The model under review builds one solid part; all positions refer to its coordinate system, in mm. A direction names the side the tool comes from. Give positions to 0.01 mm unless a question says otherwise; leave off trailing zeros. Write item = value, one per line.
```python
from build123d import *

# Parameters (mm, degrees)
SKETCH_1_R          = 1.6
SKETCH_1_R_2        = 2.1
SKETCH_1_R_3        = 2
EXTRUDE_1_DEPTH     = 5
SKETCH_2_R          = 2.25
CUT_EXTRUDE_2_DEPTH = 10
SKETCH_3_R          = 2.1
CUT_EXTRUDE_3_DEPTH = 27
CUT_EXTRUDE_4_DEPTH = 20
SKETCH_5_R          = 2.1
CUT_EXTRUDE_5_DEPTH = 20


with BuildPart() as part:
    # 草图1 → 凸台-拉伸1 (new body)
    with BuildSketch(Plane(origin=(0, 0, 0), x_dir=(1, 0, 0), z_dir=(0, 1, 0))):
        with BuildLine():
            Line((-43, -137), (43, -137))
            ThreePointArc((43, -137), (50.071067812, -134.071067812), (53, -127))
            Line((53, -127), (53, 132))
            ThreePointArc((53, 132), (50.071067812, 139.071067812), (43, 142))
            Line((43, 142), (-43, 142))
            ThreePointArc((-43, 142), (-50.071067812, 139.071067812), (-53, 132))
            Line((-53, 132), (-53, -127))
            ThreePointArc((-53, -127), (-50.071067812, -134.071067812), (-43, -137))
        make_face()
        with Locations((-40, 132)):
            Circle(SKETCH_1_R, mode=Mode.SUBTRACT)
        with Locations((-9, 132)):
            Circle(SKETCH_1_R, mode=Mode.SUBTRACT)
        with Locations((-9, 101)):
            Circle(SKETCH_1_R, mode=Mode.SUBTRACT)
        with Locations((-40, 101)):
            Circle(SKETCH_1_R, mode=Mode.SUBTRACT)
        with Locations((9, 101)):
            Circle(SKETCH_1_R, mode=Mode.SUBTRACT)
        with Locations((40, 101)):
            Circle(SKETCH_1_R, mode=Mode.SUBTRACT)
        with Locations((9, 132)):
            Circle(SKETCH_1_R, mode=Mode.SUBTRACT)
        with Locations((40, 132)):
            Circle(SKETCH_1_R, mode=Mode.SUBTRACT)
        with Locations((-37, -112)):
            Circle(SKETCH_1_R_2, mode=Mode.SUBTRACT)
        with Locations((-37, -32)):
            Circle(SKETCH_1_R_2, mode=Mode.SUBTRACT)
        with Locations((-37, 48)):
            Circle(SKETCH_1_R_2, mode=Mode.SUBTRACT)
        with Locations((37, -112)):
            Circle(SKETCH_1_R_2, mode=Mode.SUBTRACT)
        with Locations((37, -32)):
            Circle(SKETCH_1_R_2, mode=Mode.SUBTRACT)
        with Locations((37, 48)):
            Circle(SKETCH_1_R_2, mode=Mode.SUBTRACT)
        with Locations((-40, 91)):
            Circle(SKETCH_1_R_2, mode=Mode.SUBTRACT)
        with Locations((-40, 81)):
            Circle(SKETCH_1_R_2, mode=Mode.SUBTRACT)
        with Locations((-40, 71)):
            Circle(SKETCH_1_R_2, mode=Mode.SUBTRACT)
        with Locations((-40, 61)):
            Circle(SKETCH_1_R_2, mode=Mode.SUBTRACT)
        with Locations((40, 61)):
            Circle(SKETCH_1_R_2, mode=Mode.SUBTRACT)
        with Locations((40, 71)):
            Circle(SKETCH_1_R_2, mode=Mode.SUBTRACT)
        with Locations((40, 81)):
            Circle(SKETCH_1_R_2, mode=Mode.SUBTRACT)
        with Locations((40, 91)):
            Circle(SKETCH_1_R_2, mode=Mode.SUBTRACT)
        with Locations((-42.25, -5.7)):
            Circle(SKETCH_1_R_2, mode=Mode.SUBTRACT)
        with Locations((-23.75, -5.7)):
            Circle(SKETCH_1_R_2, mode=Mode.SUBTRACT)
        with Locations((23.75, -5.7)):
            Circle(SKETCH_1_R_2, mode=Mode.SUBTRACT)
        with Locations((42.25, -5.7)):
            Circle(SKETCH_1_R_2, mode=Mode.SUBTRACT)
        with Locations((-28, 32.95)):
            Circle(SKETCH_1_R_3, mode=Mode.SUBTRACT)
        with Locations((28, 32.95)):
            Circle(SKETCH_1_R_3, mode=Mode.SUBTRACT)
        with BuildLine():
            Line((21, 91.5), (-21, 91.5))
            ThreePointArc((-21, 91.5), (-23.121320344, 90.621320344), (-24, 88.5))
            Line((-24, 88.5), (-24, 54.5))
            ThreePointArc((-24, 54.5), (-23.121320344, 52.378679656), (-21, 51.5))
            Line((-21, 51.5), (21, 51.5))
            ThreePointArc((21, 51.5), (23.121320344, 52.378679656), (24, 54.5))
            Line((24, 54.5), (24, 88.5))
            ThreePointArc((24, 88.5), (23.121320344, 90.621320344), (21, 91.5))
        make_face(mode=Mode.SUBTRACT)
        with BuildLine():
            Line((-36, 37.5), (-32, 37.5))
            ThreePointArc((-32, 37.5), (-31.292893219, 37.207106781), (-31, 36.5))
            Line((-31, 36.5), (-31, 29.5))
            ThreePointArc((-31, 29.5), (-31.292893219, 28.792893219), (-32, 28.5))
            Line((-32, 28.5), (-36, 28.5))
            ThreePointArc((-36, 28.5), (-36.707106781, 28.792893219), (-37, 29.5))
            Line((-37, 29.5), (-37, 36.5))
            ThreePointArc((-37, 36.5), (-36.707106781, 37.207106781), (-36, 37.5))
        make_face(mode=Mode.SUBTRACT)
        with BuildLine():
            Line((-16, 37.5), (-12, 37.5))
            ThreePointArc((-12, 37.5), (-11.292893219, 37.207106781), (-11, 36.5))
            Line((-11, 36.5), (-11, 29.5))
            ThreePointArc((-11, 29.5), (-11.292893219, 28.792893219), (-12, 28.5))
            Line((-12, 28.5), (-16, 28.5))
            ThreePointArc((-16, 28.5), (-16.707106781, 28.792893219), (-17, 29.5))
            Line((-17, 29.5), (-17, 36.5))
            ThreePointArc((-17, 36.5), (-16.707106781, 37.207106781), (-16, 37.5))
        make_face(mode=Mode.SUBTRACT)
        with BuildLine():
            Line((37, 36.5), (37, 29.5))
            ThreePointArc((37, 29.5), (36.707106781, 28.792893219), (36, 28.5))
            Line((36, 28.5), (32, 28.5))
            ThreePointArc((32, 28.5), (31.292893219, 28.792893219), (31, 29.5))
            Line((31, 29.5), (31, 36.5))
            ThreePointArc((31, 36.5), (31.292893219, 37.207106781), (32, 37.5))
            Line((32, 37.5), (36, 37.5))
            ThreePointArc((36, 37.5), (36.707106781, 37.207106781), (37, 36.5))
        make_face(mode=Mode.SUBTRACT)
        with BuildLine():
            Line((17, 36.5), (17, 29.5))
            ThreePointArc((17, 29.5), (16.707106781, 28.792893219), (16, 28.5))
            Line((16, 28.5), (12, 28.5))
            ThreePointArc((12, 28.5), (11.292893219, 28.792893219), (11, 29.5))
            Line((11, 29.5), (11, 36.5))
            ThreePointArc((11, 36.5), (11.292893219, 37.207106781), (12, 37.5))
            Line((12, 37.5), (16, 37.5))
            ThreePointArc((16, 37.5), (16.707106781, 37.207106781), (17, 36.5))
        make_face(mode=Mode.SUBTRACT)
    extrude(amount=EXTRUDE_1_DEPTH)

    # 草图2 → 切除-拉伸2 (cut)
    with BuildSketch(Plane(origin=(0, 0, 0), x_dir=(1, 0, 0), z_dir=(0, 1, 0))):
        with Locations((-43.25, -80.8)):
            Circle(SKETCH_2_R)
        with Locations((43.25, -80.8)):
            Circle(SKETCH_2_R)
        with Locations((-43.25, -18.8)):
            Circle(SKETCH_2_R)
        with Locations((43.25, -18.8)):
            Circle(SKETCH_2_R)
    extrude(amount=CUT_EXTRUDE_2_DEPTH, mode=Mode.SUBTRACT)

    # 草图3 → 切除-拉伸3 (cut)
    with BuildSketch(Plane(origin=(0, 0, 0), x_dir=(1, 0, 0), z_dir=(0, 1, 0))):
        with Locations((2.28, -125.5)):
            Circle(SKETCH_3_R)
        with Locations((48.28, -125.5)):
            Circle(SKETCH_3_R)
        with Locations((24.28, -99.327742623)):
            Circle(SKETCH_3_R)
        with BuildLine():
            Line((37.78, -120.8), (41.78, -120.8))
            ThreePointArc((41.78, -120.8), (42.487106781, -121.092893219), (42.78, -121.8))
            Line((42.78, -121.8), (42.78, -128.8))
            ThreePointArc((42.78, -128.8), (42.487106781, -129.507106781), (41.78, -129.8))
            Line((41.78, -129.8), (37.78, -129.8))
            ThreePointArc((37.78, -129.8), (37.072893219, -129.507106781), (36.78, -128.8))
            Line((36.78, -128.8), (36.78, -121.8))
            ThreePointArc((36.78, -121.8), (37.072893219, -121.092893219), (37.78, -120.8))
        make_face()
        with BuildLine():
            Line((7.78, -120.8), (11.78, -120.8))
            ThreePointArc((11.78, -120.8), (12.487106781, -121.092893219), (12.78, -121.8))
            Line((12.78, -121.8), (12.78, -128.8))
            ThreePointArc((12.78, -128.8), (12.487106781, -129.507106781), (11.78, -129.8))
            Line((11.78, -129.8), (7.78, -129.8))
            ThreePointArc((7.78, -129.8), (7.072893219, -129.507106781), (6.78, -128.8))
            Line((6.78, -128.8), (6.78, -121.8))
            ThreePointArc((6.78, -121.8), (7.072893219, -121.092893219), (7.78, -120.8))
        make_face()
        with BuildLine():
            Line((21.28, -106.8), (27.28, -106.8))
            ThreePointArc((27.28, -106.8), (27.987106781, -107.092893219), (28.28, -107.8))
            Line((28.28, -107.8), (28.28, -111.8))
            ThreePointArc((28.28, -111.8), (27.987106781, -112.507106781), (27.28, -112.8))
            Line((27.28, -112.8), (21.28, -112.8))
            ThreePointArc((21.28, -112.8), (20.572893219, -112.507106781), (20.28, -111.8))
            Line((20.28, -111.8), (20.28, -107.8))
            ThreePointArc((20.28, -107.8), (20.572893219, -107.092893219), (21.28, -106.8))
        make_face()
        with BuildLine():
            Line((21.28, -86.8), (27.28, -86.8))
            ThreePointArc((27.28, -86.8), (27.987106781, -87.092893219), (28.28, -87.8))
            Line((28.28, -87.8), (28.28, -91.8))
            ThreePointArc((28.28, -91.8), (27.987106781, -92.507106781), (27.28, -92.8))
            Line((27.28, -92.8), (21.28, -92.8))
            ThreePointArc((21.28, -92.8), (20.572893219, -92.507106781), (20.28, -91.8))
            Line((20.28, -91.8), (20.28, -87.8))
            ThreePointArc((20.28, -87.8), (20.572893219, -87.092893219), (21.28, -86.8))
        make_face()
        with BuildLine():
            Line((-8.22, -121.8), (-8.22, -128.8))
            ThreePointArc((-8.22, -128.8), (-8.512893219, -129.507106781), (-9.22, -129.8))
            Line((-9.22, -129.8), (-13.22, -129.8))
            ThreePointArc((-13.22, -129.8), (-13.927106781, -129.507106781), (-14.22, -128.8))
            Line((-14.22, -128.8), (-14.22, -121.8))
            ThreePointArc((-14.22, -121.8), (-13.927106781, -121.092893219), (-13.22, -120.8))
            Line((-13.22, -120.8), (-9.22, -120.8))
            ThreePointArc((-9.22, -120.8), (-8.512893219, -121.092893219), (-8.22, -121.8))
        make_face()
    extrude(amount=CUT_EXTRUDE_3_DEPTH, mode=Mode.SUBTRACT)

    # 草图4 → 切除-拉伸4 (cut)
    with BuildSketch(Plane(origin=(0, 0, 0), x_dir=(1, 0, 0), z_dir=(0, 1, 0))):
        with BuildLine():
            Line((36, -95), (42, -95))
            ThreePointArc((42, -95), (44.121320344, -95.878679656), (45, -98))
            Line((45, -98), (45, -104))
            ThreePointArc((45, -104), (44.121320344, -106.121320344), (42, -107))
            Line((42, -107), (36, -107))
            ThreePointArc((36, -107), (33.878679656, -106.121320344), (33, -104))
            Line((33, -104), (33, -98))
            ThreePointArc((33, -98), (33.878679656, -95.878679656), (36, -95))
        make_face()
    extrude(amount=CUT_EXTRUDE_4_DEPTH, mode=Mode.SUBTRACT)

    # 草图5 → 切除-拉伸5 (cut)
    with BuildSketch(Plane(origin=(0, 0, 0), x_dir=(1, 0, 0), z_dir=(0, 1, 0))):
        with Locations((0, -2)):
            Circle(SKETCH_5_R)
        with Locations((-8, -102)):
            Circle(SKETCH_5_R)
        with Locations((8, -102)):
            Circle(SKETCH_5_R)
    extrude(amount=CUT_EXTRUDE_5_DEPTH, mode=Mode.SUBTRACT)


solid = part.part
```
1. Draft analysis for pull direction Z (two halves, no side actions). For faces 3 (the flat face through (24, 2, 106.8)), 4 (the flat face through (-53, 2, -4)), state which applies: +Z half, -Z half, draft (parallel to the pull), parting line (faces both ways), or undercut.
Findings below:
face_3 = undercut
face_4 = draft
2. Machinability: for faces 1 (the flat face through (24, 2, -71)), 2 (the flat face through (53, 2, -1)), which of the approach directions +Z, -Z, +X, -X, +Y, -Y give a long, thin tool a straight path to every point of the face, cutting with its end or side? Answer none if there is none.
Findings below:
face_1 = +Y, -Y
face_2 = +Z, -Z, +X, +Y, -Y
3. Insertion check: P1, Ø8, axis at x = -4.5, z = 41, coming from the -Y side; P2, Ø2.5, axis at x = 40, z = -71, coming from the +Y side. Each pin has a flat end and moves straight along its axis. Give the tip position at first contact, or say it passes through.
Findings below:
P1 = 0
P2 = through
4. Take a section at A-A on y = 0.75. Count the separate pieces of the cut face and the enclosed holes in it, and give its area (3 significant figures).
Findings below:
separate_pieces = 1
enclosed_holes = 49
area = 26,500 mm²
5. For line 1 (X direction, y = 4.15, z = -35); line 2 (Z direction, x = 13, y = 3.75); line 3 (X direction, y = 1.4, z = -48), list the stretches that pass through material, from the lowest coordinate up. Write a range as from..to.
Findings below:
line_1 = -53..-37, -31..-17, -11..11, 17..31, 37..53
line_2 = -142..-91.5, -51.5..-37.5, -28.5..137
line_3 = -53..-39.1, -34.9..34.9, 39.1..53
